Geometry check sheet. Reference: the model listing, model coordinates, mm. A direction names the side the tool comes from. Round coordinates to 2 decimals unless told otherwise and drop trailing zeros. Loops run counter-clockwise (first coordinate to the right, second up) from the corner with the lowest first, then second, coordinate; pieces in that order, holes last. Notation, with made-up numbers: (25.25, 88.5) -> (45.25, 88.5) arc R26 cw to (45.25, 126.5) -> close; hole circle Ø7 at (37, -21). An arc over 180 degrees is marked (long way). Use a Markdown table: item, result. Add a question column.
Q1. Sectioned sample at A-A, the plane x = 20. Enter the section's corners in (y, z).
Q2. Sectioned sample at B-B, the plane y = 2.5. Enter the section's corners in (x, z).
Q3. Material ranges on L1, parallel to Z at x = 7, y = 5.5; L2, parallel to Z at x = 36, y = -9.5; L3, parallel to X at y = -2.5, z = -47.5, recorded low to high.
Q4. Gauge pin test, flat ends, axial feed: P1, Ø10, axis at x = 9.5, z = -105, coming from the +Y side; P2, Ø1.5, axis at x = 26, y = -12.5, coming from the +Z side; P3, Ø4, axis at x = 27, z = -104.5, coming from the -Y side; P4, Ø9, axis at x = 20, z = 39.92, coming from the -Y side. Record the tip position at first contact, or that the pin passes through.
Q5. Sectioned sample at D-D, the plane x = 6. Enter the section's corners in (y, z), then the cut area to 3 significant figures.
Q6. Release check for a two-part mould opening along X. For faces 1 (the face through (20, 7, -16.24)), 2 (the face through (0, -1, -49)), 3 (the face through (40, -1, -49)), 4 (the face through (17, 1.3, -51.5)) record: released by +X, released by -X, zero draft, split by the parting line, or undercut.
Q7. Set-up check for faces 5 (the face through (20, -11, -53)), 6 (the face through (20, 7, -111.24)), 7 (the face through (15, -11, 43)), 8 (the face through (20, 13.24, 32)), 9 (the face through (15, -11, -138)): record each of +Z, -Z, +X, -X, +Y, -Y from which the full face is reachable in a straight line by a thin tool's end or side.
Q8. Sectioned sample at C-C, the plane y = -20. Enter the section's corners in (x, z).
```python
from build123d import *

# Parameters (mm, degrees)
BOSS_EXTRUDE1_DEPTH = 40
CUT_EXTRUDE1_REACH  = 161.395
SKETCH3_R           = 5


with BuildPart() as part:
    # Sketch2 → Boss-Extrude1 (new body)
    with BuildSketch(Plane(origin=(0, 0, 0), x_dir=(0, 0, -1), z_dir=(1, 0, 0))):
        with BuildLine():
            Line((-24.920224718, -11), (-54.920224718, -11))
            Line((-54.920224718, -11), (-54.920224718, 0))
            Line((-54.920224718, 0), (-54.920224718, 13.24))
            Line((-54.920224718, 13.24), (-16.24, 13.24))
            Line((-16.24, 13.24), (-16.24, 0))
            ThreePointArc((-16.24, 0), (0, -16.24), (16.24, 0))
            Line((16.24, 0), (16.24, 13.24))
            Line((16.24, 13.24), (78.76, 13.24))
            Line((78.76, 13.24), (78.76, 0))
            ThreePointArc((78.76, 0), (95, -16.24), (111.24, 0))
            Line((111.24, 0), (111.24, 13.24))
            Line((111.24, 13.24), (149.920224718, 13.24))
            Line((149.920224718, 13.24), (149.920224718, 0))
            Line((149.920224718, 0), (149.920224718, -11))
            Line((149.920224718, -11), (119.920224718, -11))
            ThreePointArc((119.920224718, -11), (95, -23.24), (70.079775282, -11))
            Line((70.079775282, -11), (24.920224718, -11))
            ThreePointArc((24.920224718, -11), (0, -23.24), (-24.920224718, -11))
        make_face()
    extrude(amount=BOSS_EXTRUDE1_DEPTH)

    # Sketch3 → Cut-Extrude1 (cut, up to next)
    with BuildSketch(Plane(origin=(0, 13.24, 0), x_dir=(1, 0, 0), z_dir=(0, 1, 0)), mode=Mode.PRIVATE) as cut_extrude1_sk1:
        with Locations(Location((20, -39.920224718, 0), (0, 0, 270))):
            Circle(SKETCH3_R)
    cut_extrude1_tool1 = extrude(cut_extrude1_sk1.sketch, amount=-CUT_EXTRUDE1_REACH, mode=Mode.PRIVATE) & part.part
    # Sketch3 → Cut-Extrude1 (cut, up to next)
    with BuildSketch(Plane(origin=(0, 13.24, 0), x_dir=(1, 0, 0), z_dir=(0, 1, 0)), mode=Mode.PRIVATE) as cut_extrude1_sk2:
        with Locations(Location((20, 134.920224718, 0), (0, 0, 270))):
            Circle(SKETCH3_R)
    cut_extrude1_tool2 = extrude(cut_extrude1_sk2.sketch, amount=-CUT_EXTRUDE1_REACH, mode=Mode.PRIVATE) & part.part
    # Sketch3 → Cut-Extrude1 (cut, up to next)
    with BuildSketch(Plane(origin=(0, 13.24, 0), x_dir=(1, 0, 0), z_dir=(0, 1, 0)), mode=Mode.PRIVATE) as cut_extrude1_sk3:
        with Locations(Location((20, 47.5, 0), (0, 0, 270))):
            Circle(SKETCH3_R)
    cut_extrude1_tool3 = extrude(cut_extrude1_sk3.sketch, amount=-CUT_EXTRUDE1_REACH, mode=Mode.PRIVATE) & part.part
    add(cut_extrude1_tool1.solids().sort_by_distance((20, 13.24, 39.920225))[0], mode=Mode.SUBTRACT)
    add(cut_extrude1_tool2.solids().sort_by_distance((20, 13.24, -134.920225))[0], mode=Mode.SUBTRACT)
    add(cut_extrude1_tool3.solids().sort_by_distance((20, 13.24, -47.5))[0], mode=Mode.SUBTRACT)


solid = part.part
```
Values:
| question | item | result |
|---|---|---|
| 1 | outline | (-11, -149.92) -> (13.24, -149.92) -> (13.24, -139.92) -> (-11, -139.92) -> close; (-11, -129.92) -> (13.24, -129.92) -> (13.24, -111.24) -> (0, -111.24) arc R16.24 cw to (0, -78.76) -> (13.24, -78.76) -> (13.24, -52.5) -> (-11, -52.5) -> (-11, -70.08) arc R31.49 ccw to (-11, -119.92) -> close; (-11, -42.5) -> (13.24, -42.5) -> (13.24, -16.24) -> (0, -16.24) arc R16.24 cw to (0, 16.24) -> (13.24, 16.24) -> (13.24, 34.92) -> (-11, 34.92) -> (-11, 24.92) arc R31.49 ccw to (-11, -24.92) -> close; (-11, 44.92) -> (13.24, 44.92) -> (13.24, 54.92) -> (-11, 54.92) -> close |
| 2 | outline | (0, -149.92) -> (40, -149.92) -> (40, -111.24) -> (0, -111.24) -> close; (0, -78.76) -> (40, -78.76) -> (40, -16.24) -> (0, -16.24) -> close; (0, 16.24) -> (40, 16.24) -> (40, 54.92) -> (0, 54.92) -> close; hole circle Ø10 at (20, -134.92); hole circle Ø10 at (20, -47.5); hole circle Ø10 at (20, 39.92) |
| 3 | L1 | -149.92 to -111.24, -78.76 to -16.24, 16.24 to 54.92 |
| 3 | L2 | -149.92 to -108.17, -81.83 to -13.17, 13.17 to 54.92 |
| 3 | L3 | 0 to 15, 25 to 40 |
| 4 | P1 | y = -6.22 |
| 4 | P2 | z = 24.32 |
| 4 | P3 | y = -22.33 |
| 4 | P4 | through |
| 5 | outline | (-11, -149.92) -> (13.24, -149.92) -> (13.24, -111.24) -> (0, -111.24) arc R16.24 cw to (0, -78.76) -> (13.24, -78.76) -> (13.24, -16.24) -> (0, -16.24) arc R16.24 cw to (0, 16.24) -> (13.24, 16.24) -> (13.24, 54.92) -> (-11, 54.92) -> (-11, 24.92) arc R31.49 ccw to (-11, -24.92) -> (-11, -70.08) arc R31.49 ccw to (-11, -119.92) -> close |
| 5 | area | 4,130 mm^2 |
| 6 | face 1 | zero draft |
| 6 | face 2 | released by -X |
| 6 | face 3 | released by +X |
| 6 | face 4 | undercut |
| 7 | face 5 | +X, -X, -Y |
| 7 | face 6 | +X, -X, +Y |
| 7 | face 7 | +Z, +X, -X, -Y |
| 7 | face 8 | +Z, -Z, +X, -X, +Y |
| 7 | face 9 | -Z, +X, -X, -Y |
| 8 | outline | (0, -108.91) -> (40, -108.91) -> (40, -81.09) -> (0, -81.09) -> close; (0, -13.91) -> (40, -13.91) -> (40, 13.91) -> (0, 13.91) -> close |
